Geometry: see drawing. Coordinates: mm, zero at the bounding-box minimum. A direction names the side the tool comes from. Give positions to 0.01 mm unless a question says otherwise; leave off trailing zeros. Write each loop counter-clockwise with the first axis right and the second up, starting at its lowest first coordinate (ties: lowest second). Pieces come first, ordered by that corner, then holes. Notation, with made-up numbers: (-37, 67.25) - (-31, 67.25) arc R17 cw to (-31, 77.25) - close; hole circle Ø4 at (13, 88). An arc over 180 degrees is marked (long way). Return JSON: item names as keys, results as strings.
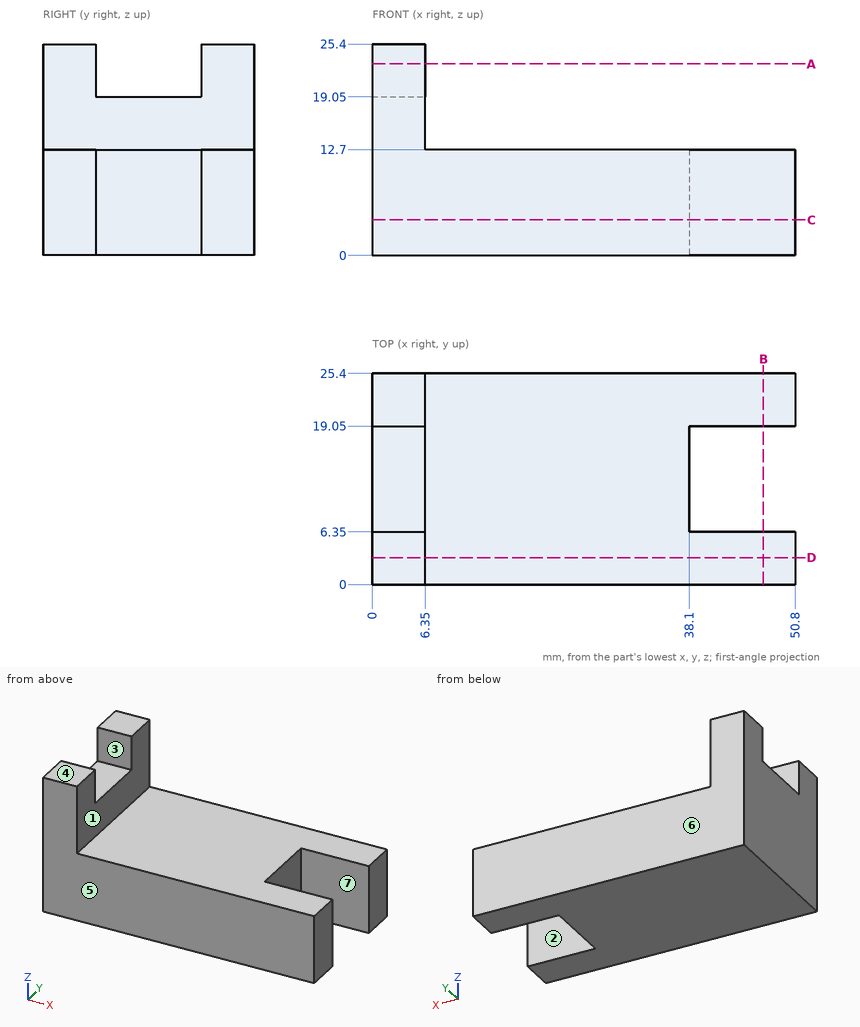
Q1. Material intervals for probe 1 along Y at (x, z) = (5.5, 23); probe 2 along Z at (x, y) = (26.5, 15.25); probe 3 along X at (y, z) = (3.25, 22), sorted ascending. Write a range as [from, to].
Answer key:
{"probe 1": "y = [0, 6.35], [19.05, 25.4]", "probe 2": "z = [0, 12.7]", "probe 3": "x = [0, 6.35]"}
Q2. Section query C-C, the plane z = 4.25. Return the cut outline in (x, y).
Answer key:
{"outline": "(0, 0) - (50.8, 0) - (50.8, 6.35) - (38.1, 6.35) - (38.1, 19.05) - (50.8, 19.05) - (50.8, 25.4) - (0, 25.4) - close"}
Q3. Pin query (flat end, axial travel): P1, Ø10, axis at x = 47, z = 6.5, coming from the -Y side; P2, Ø1, axis at x = 24, y = 16, coming from the +Z side; P3, Ø6, axis at x = 43, y = 10.5, coming from the -Z side; P4, Ø1.9, axis at x = 2, y = 12.5, coming from the +Z side. Return the tip coordinate at first contact, or that it passes through.
Answer key:
{"P1": "stops at y = 0", "P2": "stops at z = 12.7", "P3": "passes through", "P4": "stops at z = 19.05"}
Q4. Section query D-D, the plane y = 3.25. Return the cut outline in (x, z).
Answer key:
{"outline": "(0, 0) - (50.8, 0) - (50.8, 12.7) - (6.35, 12.7) - (6.35, 25.4) - (0, 25.4) - close"}
Q5. Mould query, pull axis Y, two halves, no side actions, for the marked faces 4, 5, 6 and 7. Classes: pulls with the +Y half, pulls with the -Y half, needs draft (parallel to the pull), parting line crosses it, or undercut.
Answer key:
{"face 4": "needs draft", "face 5": "pulls with the -Y half", "face 6": "pulls with the +Y half", "face 7": "undercut"}
Q6. Set-up query: the marked faces 1, 2 and 3. Return all of +Z, -Z, +X, -X, +Y, -Y with unobstructed straight access to the full face (end or side cutting, diameter ignored); none if empty.
Answer key:
{"face 1": "+Z, +X, +Y, -Y", "face 2": "+Z, -Z, +X", "face 3": "+Z, +X, -X"}
Q7. Section query B-B, the plane x = 47. Return the cut outline in (y, z), plus the area to 3 significant figures.
Answer key:
{"outline": "(0, 0) - (6.35, 0) - (6.35, 12.7) - (0, 12.7) - close; (19.05, 0) - (25.4, 0) - (25.4, 12.7) - (19.05, 12.7) - close", "area": "161 mm^2"}
Q8. Section query A-A, the plane z = 23. Return the cut outline in (x, y).
Answer key:
{"outline": "(0, 0) - (6.35, 0) - (6.35, 6.35) - (0, 6.35) - close; (0, 19.05) - (6.35, 19.05) - (6.35, 25.4) - (0, 25.4) - close"}
